Can you work these out from the model? Positions are in its coordinate system, mm. A direction names the side the tool comes from. Coordinates: 2 decimals unless noted, no trailing zeros. Order: outer loops, then holes, each group sorted by start corner. A loop starts at its lowest first (then second) coordinate and runs counter-clockwise, first axis right, second up. Notation, with made-up numbers: (20.25, -24) -> (76.25, -24) arc R17 cw to (76.25, -9) -> close; hole circle Ø2 at (89.5, -25). An arc over 180 degrees is marked (long way). Answer in a Markdown table with one row per item.
```python
from build123d import *

# Parameters (mm, degrees)
F1_DEPTH       = 68
F3_D           = 8.5
F3_CBORE_D     = 19
F3_CBORE_DEPTH = 8
F5_D           = 13.1
F7_D           = 8


with BuildPart() as f1:
    # F0 (on Top) → F1 (new body)
    with BuildSketch(Plane.XY):
        Polygon((66.851603, 12.029409), (66.851603, 38.029409), (-48.148397, 38.029409), (-48.148397, -33.970591), (66.851603, -33.970591), (66.851603, -7.970591), (-36.148397, -7.970591), (-36.148397, 12.029409), align=None)
    extrude(amount=F1_DEPTH)

    # F3 (through all)
    with Locations(Plane.XY.offset(68)):
        with Locations((20.851603, 24.943848), (20.851603, -21.056152)):
            CounterBoreHole(F3_D / 2, F3_CBORE_D / 2, F3_CBORE_DEPTH)

    # F5 (through all)
    with Locations(Plane.XZ.offset(33.970591)):
        with Locations((4.851603, 37)):
            Hole(F5_D / 2)

    # F7 (through all)
    with Locations(Plane.XZ.offset(33.970591)):
        with Locations((-25.148397, 52)):
            Hole(F7_D / 2)


solid = f1.part
```
(1) Suppose I cut it at D-D (x = -22.5). Please give me the cut outline in (y, z), and give its area (3 significant figures).
Response values:
| item | result |
|---|---|
| outline | (-33.97, 0) -> (-7.97, 0) -> (-7.97, 49) -> (-33.97, 49) -> close; (-33.97, 55) -> (-7.97, 55) -> (-7.97, 68) -> (-33.97, 68) -> close; (12.03, 0) -> (38.03, 0) -> (38.03, 49) -> (12.03, 49) -> close; (12.03, 55) -> (38.03, 55) -> (38.03, 68) -> (12.03, 68) -> close |
| area | 3,220 mm2 |
(2) I need wall thicknesses on line 1 (Y direction, x = 48, z = 14); line 2 (Y direction, x = 19.5, z = 54); line 3 (X direction, y = -21.5, z = 34.5). Which ranges of each line are inside material? Lowest first, please. Write a range as [from, to].
Response values:
| item | result |
|---|---|
| line 1 | [-33.97, -7.97], [12.03, 38.03] |
| line 2 | [-33.97, -25.09], [-17.03, -7.97], [12.03, 20.91], [28.97, 38.03] |
| line 3 | [-48.15, -1.2], [10.91, 16.62], [25.08, 66.85] |
(3) Suppose I cut it at B-B (x = 45.5). Please give me the cut outline in (y, z), and give its area (3 significant figures).
Response values:
| item | result |
|---|---|
| outline | (-33.97, 0) -> (-7.97, 0) -> (-7.97, 68) -> (-33.97, 68) -> close; (12.03, 0) -> (38.03, 0) -> (38.03, 68) -> (12.03, 68) -> close |
| area | 3,540 mm2 |
(4) Will these pins go through, and if not, where does the flat tip stop? pin 1 Ø15 at (x, y) = (20.85, 24.94) entering from -Z; pin 2 Ø8 at (x, z) = (4.85, 37) entering from -Y; pin 3 Ø5.5 at (x, y) = (23.5, -16.5) entering from +Z; pin 4 Ø10 at (y, z) = (3.5, 48.5) entering from +X.
Response values:
| item | result |
|---|---|
| pin 1 | z = 0 |
| pin 2 | through |
| pin 3 | z = 60 |
| pin 4 | x = -36.15 |
(5) On a 3-axis mill with a long thin cutter (end or side, diameter ignored), from which of +Z, -Z, +X, -X, +Y, -Y can I reach the whole of each face in a straight line? I mean faces 1 (the flat face through (-36.148, 2, 34)), 2 (the flat face through (9, 19, 0)), 3 (the flat face through (23, 21, 60)). Say none if no direction works.
Response values:
| item | result |
|---|---|
| face 1 | +Z, -Z, +X |
| face 2 | -Z, +X, -X, +Y, -Y |
| face 3 | +Z |
(6) We'd pull the mould along X, two halves only. Please class faces 4 (the cylindrical face through (24.224, 22.358, 29.58)), 5 (the cylindrical face through (13.313, -26.837, 64.056)), 6 (the flat face through (9, -33.971, 26)), 7 (the flat face through (66.852, -21, 34)): +X half, -X half, draft (parallel to the pull), parting line (faces both ways), or undercut.
Response values:
| item | result |
|---|---|
| face 4 | undercut |
| face 5 | undercut |
| face 6 | draft |
| face 7 | +X half |
(7) Suppose I cut it at A-A (z = 37). Please give me the cut outline in (x, y), and give its area (3 significant figures).
Response values:
| item | result |
|---|---|
| outline | (-48.15, -33.97) -> (-1.7, -33.97) -> (-1.7, -7.97) -> (-36.15, -7.97) -> (-36.15, 12.03) -> (-1.7, 12.03) -> (-1.7, 38.03) -> (-48.15, 38.03) -> close; (11.4, -33.97) -> (66.85, -33.97) -> (66.85, -7.97) -> (11.4, -7.97) -> close; (11.4, 12.03) -> (66.85, 12.03) -> (66.85, 38.03) -> (11.4, 38.03) -> close; hole circle Ø8.5 at (20.85, -21.06); hole circle Ø8.5 at (20.85, 24.94) |
| area | 5,430 mm2 |
(8) Suppose I cut it at C-C (y = -28). Please give me the cut outline in (x, z).
Response values:
| item | result |
|---|---|
| outline | (-48.15, 0) -> (66.85, 0) -> (66.85, 68) -> (27.33, 68) -> (27.33, 60) -> (14.37, 60) -> (14.37, 68) -> (-48.15, 68) -> close; hole circle Ø8 at (-25.15, 52); hole circle Ø13.1 at (4.85, 37) |
